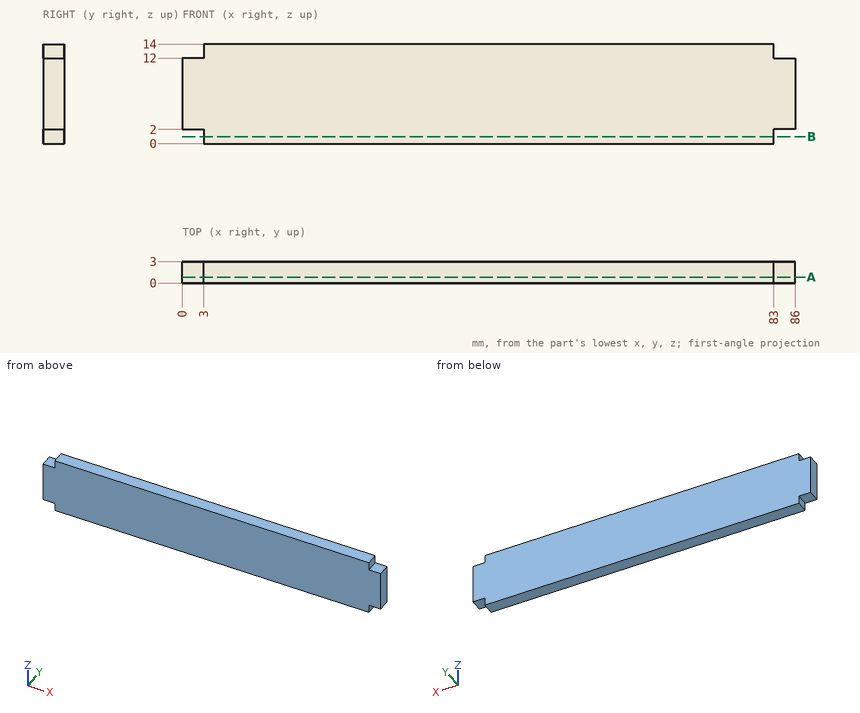
Geometry: see drawing. Coordinates: mm, zero at the bounding-box minimum. Round coordinates to 2 decimals unless told otherwise and drop trailing zeros. Loops run counter-clockwise (first coordinate to the right, second up) from the corner with the lowest first, then second, coordinate; pieces in that order, holes last. Notation, with made-up numbers: M 44.25,-21 L 68.25,-21 A14 cw 68.25,6 Z; hole C 13,-25.5 d6. An arc over 180 degrees is marked long. Use a Markdown table: item, result. Add a question column.
1. Contact query for flat-ended pins moving along their axis: P1, Ø1, axis at y = 1, z = 0.5, coming from the +X side; P2, Ø0.6, axis at y = 2, z = 1, coming from the -X side; P3, Ø0.9, axis at x = 1, y = 1, coming from the +Z side. Output: stop coordinate, or through.
2. Line query: line 1 (X direction, y = 2.2, z = 1.75). Output: solid intervals per line, ascending.
3. Section query B-B on z = 1. Return the cut outline in (x, y).
4. Section query A-A on y = 0.85. Return the cut outline in (x, z), then the cut area to 3 significant figures.
Reported:
| question | item | result |
|---|---|---|
| 1 | P1 | stops at x = 83 |
| 1 | P2 | stops at x = 3 |
| 1 | P3 | stops at z = 12 |
| 2 | line 1 | x = 3 to 83 |
| 3 | outline | M 3,0 L 83,0 L 83,3 L 3,3 Z |
| 4 | outline | M 0,2 L 3,2 L 3,0 L 83,0 L 83,2 L 86,2 L 86,12 L 83,12 L 83,14 L 3,14 L 3,12 L 0,12 Z |
| 4 | area | 1,180 mm² |
